Build history of the part. All positions in model axes, mm. A direction names the side the tool comes from. Give positions to 0.01 mm unless a question says otherwise; leave off trailing zeros. Order: outer loops, then holes, each group sorted by start corner. A loop starts at its lowest first (then second) coordinate and runs counter-clockwise, first axis right, second up. Notation, with made-up numbers: M -4.5,-38 L 47.5,-38 A9 ccw 47.5,-31 Z; hole C 49.5,56.5 d1. An arc over 180 degrees is marked long. One line per item, written item: value.
from build123d import *

# Parameters (mm, degrees)
F0_W     = 300
F0_H     = 200
F1_DEPTH = 5
F2_W     = 300
F2_H     = 15
F2_H_2   = 5
F3_DEPTH = 150


with BuildPart() as f1:
    # F0 (on Front) → F1 (new body)
    with BuildSketch(Plane.XZ):
        Rectangle(F0_W, F0_H)
    extrude(amount=F1_DEPTH)

    # F2 (on face) → F3 (join)
    with BuildSketch(Plane(origin=(0, 0, 0), x_dir=(-1, 0, 0), z_dir=(0, 1, 0))):
        with Locations((0, 92.5)):
            Rectangle(F2_W, F2_H)
        with Locations((0, -57.5)):
            Rectangle(F2_W, F2_H)
        with Locations((0, -97.5)):
            Rectangle(F2_W, F2_H_2)
    extrude(amount=F3_DEPTH)


solid = f1.part
1) Tool access for faces 4 (the face through (2, 74, -95)), 5 (the face through (-2, -5, 1)): list every direction of +Z, -Z, +X, -X, +Y, -Y with a clear straight run to the whole face (end or side of a thin tool).
Check values:
face 4: +X, -X, +Y
face 5: +Z, -Z, +X, -X, -Y
2) Drill centre lines: probe 1 along Z at (x, y) = (29.5, 93.5); probe 2 along Y at (x, z) = (33, 22). Where is each one in solid material? Low to high. Write a range as from..to.
Check values:
probe 1: -100..-95, -65..-50, 85..100
probe 2: -5..0
3) Saw through at C-C, the plane z = 50.5. Write the cut outline in (x, y), then the cut area to 3 significant figures.
Check values:
outline: M -150,-5 L 150,-5 L 150,0 L -150,0 Z
area: 1,500 mm^2
4) Saw through at A-A, the plane y = 99.5. Write the cut outline in (x, z).
Check values:
outline: M -150,-100 L 150,-100 L 150,-95 L -150,-95 Z; M -150,-65 L 150,-65 L 150,-50 L -150,-50 Z; M -150,85 L 150,85 L 150,100 L -150,100 Z
5) Saw through at B-B, the plane x = 22. Write the cut outline in (y, z), then the cut area to 3 significant figures.
Check values:
outline: M -5,-100 L 150,-100 L 150,-95 L 0,-95 L 0,-65 L 150,-65 L 150,-50 L 0,-50 L 0,85 L 150,85 L 150,100 L -5,100 Z
area: 6,250 mm^2
6) Mould opens along Z. For faces 1 (the face through (2, 74, -50)), 2 (the face through (2, 150, 93)), 3 (the face through (-2, 74, -100)) say: released by +Z, released by -Z, zero draft, split by the parting line, or undercut.
Check values:
face 1: undercut
face 2: zero draft
face 3: released by -Z
7) Pin check, flat tip, straight feed: pin 1 (6 mm diameter, centred on x = 109.5, z = -28, fed in from +Y). Stop position of the tip, or through.
Check values:
pin 1: y = 0
